Work out the finished part from the listing and answer in its coordinate system (mm). Face numbers are marked on the shaded views. A direction names the side the tool comes from. Round coordinates to 2 decimals unless told otherwise and drop trailing zeros. Loops run counter-clockwise (first coordinate to the right, second up) from the corner with the lowest first, then second, coordinate; pieces in that order, holes last. Notation, with made-up numbers: (83.25, 46.5) - (131.25, 46.5) arc R16 cw to (131.25, 66.5) - close; hole circle Ø3 at (46, 2.25). An arc over 180 degrees is marked (long way). Answer as CSV lines item,"result". Start each with the question number.
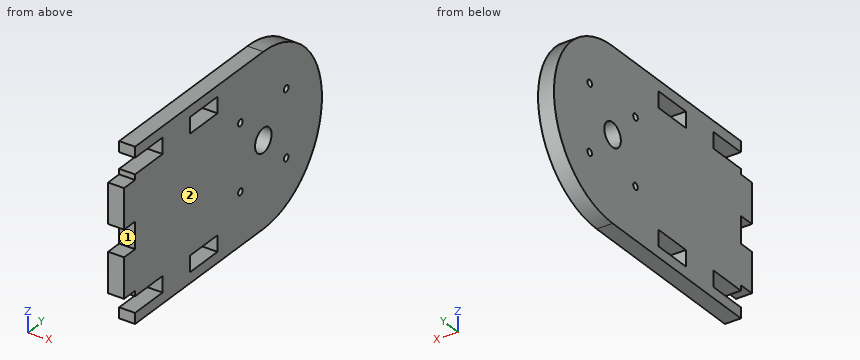
```python
from build123d import *

# Parameters (mm, degrees)
CROQUIS1_R                = 4.5
SALIENTE_EXTRUIR1_DEPTH   = 3
TALADRO_ROSCADO_M3X0_51_D = 2.5
CROQUIS6_W                = 6
CROQUIS6_H                = 15
CORTAR_EXTRUIR1_DEPTH     = 75.491610266
CROQUIS7_W                = 15
CROQUIS7_H                = 6
SALIENTE_EXTRUIR3_DEPTH   = 6


with BuildPart() as part:
    # Croquis1 → Saliente-Extruir1 (new, symmetric)
    with BuildSketch(Plane(origin=(0, 0, 0), x_dir=(0, 0, -1), z_dir=(1, 0, 0))):
        with BuildLine():
            Line((-32, -35), (-32, 35))
            ThreePointArc((-32, 35), (0, 67), (32, 35))
            Line((32, 35), (32, -35))
            Line((32, -35), (-32, -35))
        make_face()
        with Locations((0, 35)):
            Circle(CROQUIS1_R, mode=Mode.SUBTRACT)
    extrude(amount=SALIENTE_EXTRUIR1_DEPTH, both=True)

    # Taladro roscado M3x0.51 (through all)
    with Locations(Plane(origin=(3, 0, 0), x_dir=(0, 0, -1), z_dir=(1, 0, 0))):
        with Locations((12.5, 47.5), (12.5, 22.5), (-12.5, 22.5), (-12.5, 47.5)):
            Hole(TALADRO_ROSCADO_M3X0_51_D / 2)

    # Croquis6 → Cortar-Extruir1 (cut, through all)
    with BuildSketch(Plane(origin=(3, 0, 0), x_dir=(0, 0, -1), z_dir=(1, 0, 0))):
        with Locations((-25, 2.5)):
            Rectangle(CROQUIS6_W, CROQUIS6_H)
        with Locations((-25, -27.5)):
            Rectangle(CROQUIS6_W, CROQUIS6_H)
        with Locations((25, -27.5)):
            Rectangle(CROQUIS6_W, CROQUIS6_H)
        with Locations((25, 2.5)):
            Rectangle(CROQUIS6_W, CROQUIS6_H)
    extrude(amount=-CORTAR_EXTRUIR1_DEPTH, mode=Mode.SUBTRACT)

    # Croquis7 → Saliente-Extruir3 (add, through all)
    with BuildSketch(Plane(origin=(3, 0, 0), x_dir=(0, 0, -1), z_dir=(1, 0, 0))):
        with Locations((-12.5, -38)):
            Rectangle(CROQUIS7_W, CROQUIS7_H)
        with Locations((12.5, -38)):
            Rectangle(CROQUIS7_W, CROQUIS7_H)
    extrude(amount=-SALIENTE_EXTRUIR3_DEPTH)


solid = part.part
```
Item 1: Section C-C, the plane x = -0.35 is taken. Count the separate pieces of the cut face and the enclosed holes in it, and give its area (3 significant figures).
Item 2: Section A-A, the plane y = 22.5 is taken. Give the vertices of the cut face in (x, z), and give its area (3 significant figures).
Item 3: Flat-ended cylindrical pins translate along their axes: pin 1 Ø2 at (y, z) = (47.5, 12.5) entering from +X; pin 2 Ø1.8 at (x, z) = (-1.5, 0.5) entering from -Y; pin 3 Ø3 at (x, z) = (-2, 15) entering from +Y; pin 4 Ø1.8 at (x, z) = (1, -24.5) entering from -Y. Find the tip coordinate at first contact, or state that the pin passes through.
Item 4: Find the intervals of material crossed by L1, parallel to Z at x = -0.2, y = 5; L2, parallel to Y at x = -0.8, z = 12.5; L3, parallel to Y at x = -0.45, z = -25.5, in increasing order.
Item 5: Which of the six approach directions +Z, -Z, +X, -X, +Y, -Y give full straight-line access (tool end or side, diameter ignored) to the marked faces 1 and 2?
Item 6: Section B-B, the plane z = 0 is taken. Give the vertices of the cut face in (x, y).
Item 7: Section D-D, the plane z = -12.5 is taken. Give the vertices of the cut face in (x, y).
Answer:
1,separate pieces,"1"
1,enclosed holes,"7"
1,area,"5,830 mm²"
2,outline,"(-3, -32) - (3, -32) - (3, -13.75) - (-3, -13.75) - close; (-3, -11.25) - (3, -11.25) - (3, 11.25) - (-3, 11.25) - close; (-3, 13.75) - (3, 13.75) - (3, 32) - (-3, 32) - close"
2,area,"354 mm²"
3,pin 1,"passes through"
3,pin 2,"stops at y = -35"
3,pin 3,"stops at y = 64.01"
3,pin 4,"stops at y = -20"
4,L1,"z = -32 to -28, -22 to 22, 28 to 32"
4,L2,"y = -41 to 21.25, 23.75 to 46.25, 48.75 to 64.46"
4,L3,"y = -20 to -5, 10 to 54.33"
5,face 1,"+X, -X, -Y"
5,face 2,"+Z, -Z, +X, +Y, -Y"
6,outline,"(-3, -35) - (3, -35) - (3, 30.5) - (-3, 30.5) - close; (-3, 39.5) - (3, 39.5) - (3, 67) - (-3, 67) - close"
7,outline,"(-3, -41) - (3, -41) - (3, 21.25) - (-3, 21.25) - close; (-3, 23.75) - (3, 23.75) - (3, 46.25) - (-3, 46.25) - close; (-3, 48.75) - (3, 48.75) - (3, 64.46) - (-3, 64.46) - close"
